Work out the finished part from the listing and answer in its coordinate system (mm). Face numbers are marked on the shaded views. A direction names the side the tool comes from. Give positions to 0.01 mm unless a question says otherwise; leave off trailing zeros. Loops run counter-clockwise (first coordinate to the right, second up) from the corner with the lowest first, then second, coordinate; pieces in that order, holes last.
from build123d import *

# Parameters (mm, degrees)
F0_R          = 29.8
F1_DEPTH      = 5
F3_DEPTH      = 5
F3_DEPTH_BACK = 5
F5_DEPTH      = 20
F6_DEPTH      = 23.78
F7_T2_ANGLE   = 180
F7_T4_ANGLE   = 180


# Not quite as in the source:
# - a fillet or chamfer that OpenCascade refuses, or shapes differently, is made with other operations: its cross-section is extruded or revolved along the edge and cut away or added


with BuildPart() as f1:
    # F0 (on Top) → F1 (new body)
    with BuildSketch(Plane.XY):
        Circle(F0_R)
        Polygon((0, -26.4465436339), (-3, -22.7629262954), (0, -22.7629262954), (3, -22.7629262954), align=None, mode=Mode.SUBTRACT)
    extrude(amount=F1_DEPTH)

    # F2 (on Right) → F3 (join, two sides)
    with BuildSketch(Plane.YZ) as f3_sk:
        with BuildLine():
            Line((-29.4, 5), (29.4, 5))
            ThreePointArc((29.4, 5), (0, 34.4), (-29.4, 5))
        make_face()
    extrude(amount=-F3_DEPTH)
    extrude(f3_sk.sketch, amount=F3_DEPTH_BACK)

    # F4 (on Top) → F5 (cut)
    with BuildSketch(Plane.XY):
        with BuildLine():
            ThreePointArc((-3.0525563058, 1.38), (-0.7058457252, -3.2747949267), (3.35, 0))
            ThreePointArc((3.35, 0), (3.2747949267, 0.7058457252), (3.0525563058, 1.38))
            Line((3.0525563058, 1.38), (-3.0525563058, 1.38))
        make_face()
    extrude(amount=F5_DEPTH, mode=Mode.SUBTRACT)

    # F0 (on Top) → F6 (join)
    with BuildSketch(Plane.XY):
        Polygon((0, -22.7629262954), (-3, -22.7629262954), (0, -26.4465436339), (3, -22.7629262954), align=None)
    extrude(amount=F6_DEPTH)

    # F7: fillet of radius 2 on 2 edges, made by hand

    # F7_s1 → F7_t2 (revolve, cut)
    with BuildSketch(Plane.XY.offset(5)):
        with BuildLine():
            ThreePointArc((-3, 29.4), (-4.4142135624, 28.8142135624), (-5, 27.4))
            Line((-5, 27.4), (-5, 29.4))
            Line((-5, 29.4), (-3, 29.4))
        make_face()
    revolve(axis=Axis((-5, 0, 5), (1, 0, 0)), revolution_arc=F7_T2_ANGLE, mode=Mode.SUBTRACT)

    # F7_s3 → F7_t4 (revolve, cut)
    with BuildSketch(Plane.XY.offset(5)):
        with BuildLine():
            ThreePointArc((5, 27.4), (4.4142135624, 28.8142135624), (3, 29.4))
            Line((3, 29.4), (5, 29.4))
            Line((5, 29.4), (5, 27.4))
        make_face()
    revolve(axis=Axis((5, 0, 5), (1, 0, 0)), revolution_arc=F7_T4_ANGLE, mode=Mode.SUBTRACT)


solid = f1.part
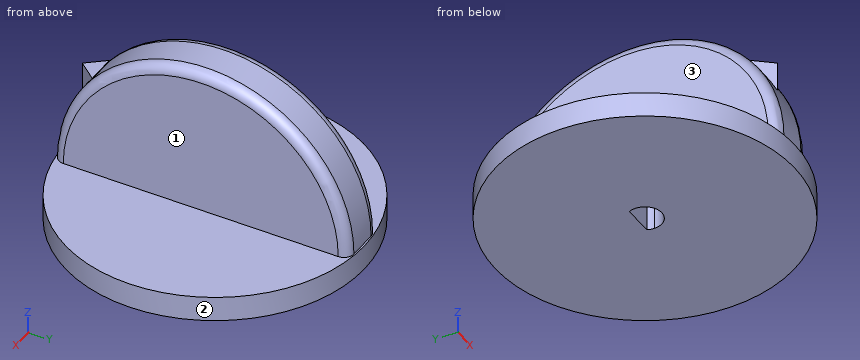
Item 1: Flat-ended cylindrical pins translate along their axes: pin 1 Ø2.5 at (x, y) = (-0.5, -1) entering from -Z; pin 2 Ø8 at (y, z) = (11, 16) entering from +X; pin 3 Ø1.5 at (y, z) = (4, 24.5) entering from -X; pin 4 Ø2 at (x, z) = (10, 7.5) entering from -Y. Find the tip coordinate at first contact, or state that the pin passes through.
Item 2: For the marked faces 1, 2 and 3, determine the directions among +Z, -Z, +X, -X, +Y, -Y from which every point of the face is accessible in a straight line to the end or side of a thin tool.
Item 3: Consider line 1 (Y direction, x = 0, z = 4.25); line 2 (X direction, y = 0, z = 7); line 3 (Z direction, x = -6, y = 0.5). Determine where each line is inside the solid, lowest interval first.
Item 4: Find section B-B, the plane x = -17.5. Write down the section's boundary in (y, z).
Item 5: Find section A-A, the plane x = -24.5. Write down the section's boundary in (y, z), plus the area to 3 significant figures.
Ans:
1. pin 1: stops at z = 20
1. pin 2: stops at x = 5
1. pin 3: stops at x = -5
1. pin 4: passes through
2. face 1: +Z, +X, +Y, -Y
2. face 2: +Z, -Z
2. face 3: +Z, -X, +Y, -Y
3. line 1: y = -29.8 to -3.35, 1.38 to 29.8
3. line 2: x = -5 to -3.35, 3.35 to 5
3. line 3: z = 0 to 5
4. outline: (-24.12, 0) - (24.12, 0) - (24.12, 5) - (-24.12, 5) - close
5. outline: (-16.96, 0) - (16.96, 0) - (16.96, 5) - (-16.96, 5) - close
5. area: 170 mm2
